The listing builds one solid part. Answer for the finished solid, in the listing's coordinates (mm). Face numbers are marked on the shaded views. A direction names the side the tool comes from. Round coordinates to 2 decimals unless told otherwise and drop trailing zeros. Write each loop counter-clockwise with the first axis right and the second up, starting at its lowest first coordinate (ties: lowest second). Pieces come first, ordered by that corner, then holes.
(1) A cutting plane is placed at A-A, the plane y = -25.25. Give the vertices of the cut face in (x, z).
(2) Each of these flat-tipped pins is pushed along its axis until it touches: pin 1 Ø4.5 at (x, y) = (-26.25, -9.25) entering from -Z; pin 2 Ø2.5 at (x, z) = (1, -4) entering from +Y; pin 3 Ø1.5 at (x, z) = (-0.5, 6) entering from +Y. Where does it stop, or does it pass through?
(3) A cutting plane is placed at C-C, the plane x = 12.5. Give the vertices of the cut face in (y, z) (3 decimals).
(4) For the marked faces 1, 2 and 3, determine the directions among +Z, -Z, +X, -X, +Y, -Y from which every point of the face is accessible in a straight line to the end or side of a thin tool.
(5) A cutting plane is placed at B-B, the plane x = -19.25. Give the vertices of the cut face in (y, z).
(6) Find the intervals of material crossed by probe 1 along Y at (x, z) = (-6.25, 5.5); probe 2 along X at (y, z) = (-12.5, 9.3); probe 3 along Y at (x, z) = (-19.25, 7.75), in increasing order.
from build123d import *

# Parameters (mm, degrees)
SKETCH2_W                      = 60
SKETCH2_H                      = 72
BOSS_EXTRUDE1_DEPTH            = 10
SKETCH9_W                      = 60
SKETCH9_H                      = 20
BOSS_EXTRUDE2_DEPTH            = 9
CBORE_FOR_M3_SHCS1_AT_2_COUNT  = 2
CBORE_FOR_M3_SHCS1_AT_2_PITCH  = 25
CBORE_FOR_M3_SHCS1_AT_3_COUNT  = 2
CBORE_FOR_M3_SHCS1_AT_3_PITCH  = 35.355339059
CBORE_FOR_M3_SHCS1_AT_4_COUNT  = 2
CBORE_FOR_M3_SHCS1_AT_4_PITCH  = 25
CUT_EXTRUDE1_DEPTH             = 11
SKETCH8_R                      = 2.1
CUT_EXTRUDE2_DEPTH             = 49.135226186
SKETCH14_W                     = 60
SKETCH14_H                     = 9.57
BOSS_EXTRUDE3_DEPTH            = 10
CBORE_FOR_M3_SHCS2_D           = 3.4
CBORE_FOR_M3_SHCS2_CBORE_D     = 6.5
CBORE_FOR_M3_SHCS2_CBORE_DEPTH = 3
CUT_EXTRUDE3_DEPTH             = 58.772181022
BOSS_EXTRUDE4_DEPTH            = 10
SKETCH20_R                     = 0.9
CUT_EXTRUDE4_DEPTH             = 10
SKETCH21_W                     = 5
SKETCH21_H                     = 7
CUT_EXTRUDE5_DEPTH             = 10


with BuildPart() as part:
    # Sketch2 → Boss-Extrude1 (new body)
    with BuildSketch(Plane.XY):
        Rectangle(SKETCH2_W, SKETCH2_H)
    extrude(amount=BOSS_EXTRUDE1_DEPTH)

    # Sketch9 → Boss-Extrude2 (add)
    with BuildSketch(Plane(origin=(0, 0, 0), x_dir=(-1, 0, 0), z_dir=(0, 0, -1))):
        with Locations((0, 26)):
            Rectangle(SKETCH9_W, SKETCH9_H)
    extrude(amount=BOSS_EXTRUDE2_DEPTH)

    # Sketch6 → CBORE for M3 SHCS1 (revolve, cut)
    with BuildSketch(Plane(origin=(-12.5, 12.5, 10), x_dir=(0, -1, 0), z_dir=(1, 0, 0))):
        Polygon((0, 0), (0, 11.021463052), (1.7, 10), (1.7, 3), (3.25, 3), (3.25, 0.025), (3.275, 0), align=None)
    cbore_for_m3_shcs1 = revolve(axis=Axis((-12.5, 12.5, 16.35), (0, 0, -1)), mode=Mode.SUBTRACT)

    # CBORE for M3 SHCS1 at 2: CBORE for M3 SHCS1 ×2
    with Locations(*[(i * CBORE_FOR_M3_SHCS1_AT_2_PITCH, 0, 0) for i in range(1, CBORE_FOR_M3_SHCS1_AT_2_COUNT)]):
        add(cbore_for_m3_shcs1, mode=Mode.SUBTRACT)

    # CBORE for M3 SHCS1 at 3: CBORE for M3 SHCS1 ×2
    with Locations(*[Vector(0.7071067811865477, -0.7071067811865475, 0) * (i * CBORE_FOR_M3_SHCS1_AT_3_PITCH) for i in range(1, CBORE_FOR_M3_SHCS1_AT_3_COUNT)]):
        add(cbore_for_m3_shcs1, mode=Mode.SUBTRACT)

    # CBORE for M3 SHCS1 at 4: CBORE for M3 SHCS1 ×2
    with Locations(*[(0, -i * CBORE_FOR_M3_SHCS1_AT_4_PITCH, 0) for i in range(1, CBORE_FOR_M3_SHCS1_AT_4_COUNT)]):
        add(cbore_for_m3_shcs1, mode=Mode.SUBTRACT)

    # Sketch7 → Cut-Extrude1 (cut)
    with BuildSketch(Plane.XY.offset(10)):
        Polygon((4.041451884, 21.5), (2.020725942, 25), (-2.020725942, 25), (-4.041451884, 21.5), (-2.020725942, 18), (2.020725942, 18), align=None)
        Polygon((4.041451884, 30.5), (2.020725942, 34), (-2.020725942, 34), (-4.041451884, 30.5), (-2.020725942, 27), (2.020725942, 27), align=None)
    extrude(amount=-CUT_EXTRUDE1_DEPTH, mode=Mode.SUBTRACT)

    # Sketch8 → Cut-Extrude2 (cut, through all)
    with BuildSketch(Plane.XY.offset(-1)):
        with Locations((0, 30.5)):
            Circle(SKETCH8_R)
        with Locations((0, 21.5)):
            Circle(SKETCH8_R)
    extrude(amount=-CUT_EXTRUDE2_DEPTH, mode=Mode.SUBTRACT)

    # Sketch14 → Boss-Extrude3 (add)
    with BuildSketch(Plane.XY.offset(10)):
        with Locations((0, -40.785)):
            Rectangle(SKETCH14_W, SKETCH14_H)
    extrude(amount=-BOSS_EXTRUDE3_DEPTH)

    # CBORE for M3 SHCS2 (through all)
    with Locations(Plane(origin=(0, 0, 0), x_dir=(-1, 0, 0), z_dir=(0, 0, -1))):
        with Locations((19.25, -25.25), (12.25, -9.25), (26.25, -9.25)):
            CounterBoreHole(CBORE_FOR_M3_SHCS2_D / 2, CBORE_FOR_M3_SHCS2_CBORE_D / 2, CBORE_FOR_M3_SHCS2_CBORE_DEPTH)

    # Sketch18 → Cut-Extrude3 (cut, through all)
    with BuildSketch(Plane.XY.offset(10)):
        Polygon((0, -45.57), (30, -15.57), (30, -45.57), align=None)
    extrude(amount=-CUT_EXTRUDE3_DEPTH, mode=Mode.SUBTRACT)

    # Sketch19 → Boss-Extrude4 (add)
    with BuildSketch(Plane.XY.offset(10)):
        Polygon((-30, 36), (-30, 65), (-4, 65), (30, 36), align=None)
    extrude(amount=-BOSS_EXTRUDE4_DEPTH)

    # Sketch20 → Cut-Extrude4 (cut)
    with BuildSketch(Plane.XY.offset(10)):
        with Locations((-27.75, 51.284)):
            Circle(SKETCH20_R)
        with Locations((-27.75, 38.584)):
            Circle(SKETCH20_R)
        with Locations((-6.25, 38.584)):
            Circle(SKETCH20_R)
        with Locations((-6.25, 51.284)):
            Circle(SKETCH20_R)
    extrude(amount=-CUT_EXTRUDE4_DEPTH, mode=Mode.SUBTRACT)

    # Sketch21 → Cut-Extrude5 (cut)
    with BuildSketch(Plane(origin=(22.785, -22.785, 0), x_dir=(0, 0, -1), z_dir=(0.707106781186544, -0.7071067811865511, 0))):
        with Locations((-7.5, -26.722856019)):
            Rectangle(SKETCH21_W, SKETCH21_H)
    extrude(amount=-CUT_EXTRUDE5_DEPTH, mode=Mode.SUBTRACT)


solid = part.part
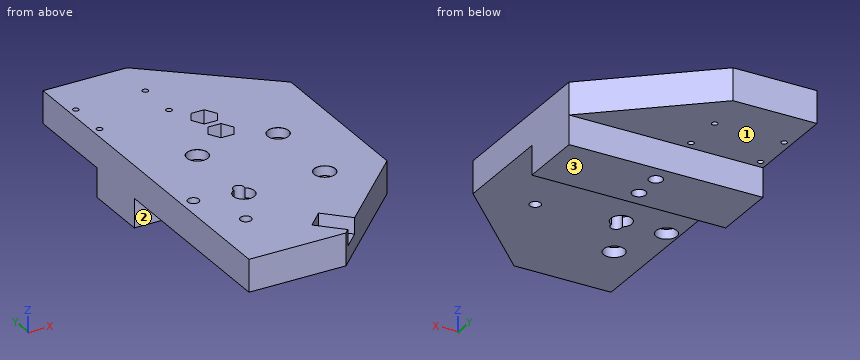
Solutions:
1. outline: (-30, 0) - (-22.5, 0) - (-22.5, 3) - (-20.95, 3) - (-20.95, 10) - (-30, 10) - close; (-17.55, 3) - (-16, 3) - (-16, 0) - (20.32, 0) - (20.32, 10) - (-17.55, 10) - close
2. pin 1: stops at z = 3
2. pin 2: stops at y = 36
2. pin 3: stops at y = 62.65
3. outline: (-33.07, 0) - (-14.2, 0) - (-14.2, 7) - (-15.75, 7) - (-15.75, 9.975) - (-15.775, 10) - (-33.07, 10) - close; (-10.8, 0) - (10.8, 0) - (10.8, 7) - (9.25, 7) - (9.25, 9.975) - (9.225, 10) - (-9.225, 10) - (-9.25, 9.975) - (-9.25, 7) - (-10.8, 7) - close; (14.2, 0) - (16, 0) - (16, -9) - (36, -9) - (36, 0) - (50.926, 0) - (50.926, 10) - (15.775, 10) - (15.75, 9.975) - (15.75, 7) - (14.2, 7) - close
4. face 1: -Z, +X, -X, +Y
4. face 2: -Z, +X, -X, -Y
4. face 3: -Z, +X, -X, +Y, -Y
5. outline: (-45.57, 0) - (-28.5, 0) - (-28.5, 3) - (-26.95, 3) - (-26.95, 10) - (-45.57, 10) - close; (-23.55, 3) - (-22, 3) - (-22, 0) - (16, 0) - (16, -9) - (36, -9) - (36, 0) - (65, 0) - (65, 10) - (-23.55, 10) - close
6. probe 1: y = -45.57 to 37.68, 39.48 to 50.38, 52.18 to 65
6. probe 2: x = -30 to -15.75, -9.25 to 9.25, 15.75 to 30
6. probe 3: y = -45.57 to -26.95, -23.55 to 65
